The listing builds one solid part. Answer for the finished solid, in the listing's coordinates (mm). A direction names the side the tool comes from. Round coordinates to 2 decimals unless told otherwise and drop trailing zeros. Write each loop counter-clockwise with the first axis right and the second up, starting at its lowest first coordinate (ties: lowest second). Pieces come first, ordered by that corner, then holes. Notation, with made-up numbers: M 43.5,5 L 73.5,5 A10 cw 73.5,19 Z; hole C 60,-9.5 d6. An arc over 180 degrees is marked long. Put each result on its own line as item: value. Start each with the question number.
```python
from build123d import *

# Parameters (mm, degrees)
SKETCH1_W               = 21.8
SKETCH1_H               = 39
BOSS_EXTRUDE1_DEPTH     = 3
BOSS_EXTRUDE2_DEPTH     = 3
BOSS_EXTRUDE4_DEPTH     = 21
SKETCH4_W               = 21.8
SKETCH4_H               = 39
BOSS_EXTRUDE5_DEPTH     = 2
CUT_EXTRUDE1_DEPTH      = 50.807730324
CUT_EXTRUDE1_DEPTH_BACK = 50.807730324
SKETCH5_W               = 14
SKETCH5_H               = 20
BOSS_EXTRUDE6_DEPTH     = 5
SKETCH7_W               = 14.6
SKETCH7_H               = 1.5
CUT_EXTRUDE2_DEPTH      = 2
SKETCH8_W               = 16.04420395
SKETCH8_H               = 34.30198165
CUT_EXTRUDE3_DEPTH      = 35.279148181
SKETCH9_W               = 16.04420395
SKETCH9_H               = 34.30198165
CUT_EXTRUDE4_DEPTH      = 2
SKETCH10_W              = 2.1
SKETCH10_H              = 1.5
CUT_EXTRUDE5_DEPTH      = 2
SKETCH11_W              = 2.1
SKETCH11_H              = 1.5
CUT_EXTRUDE6_DEPTH      = 2
SKETCH13_W              = 18.8
SKETCH13_H              = 1.5
CUT_EXTRUDE7_DEPTH      = 3
FILLET3_R               = 5
FILLET4_R               = 5
SKETCH17_W              = 1.5
SKETCH17_H              = 16
BOSS_EXTRUDE8_DEPTH     = 2
FILLET5_R               = 5
BOSS_EXTRUDE9_DEPTH     = 5
SKETCH24_R              = 2.25
BOSS_EXTRUDE10_DEPTH    = 8
BOSS_EXTRUDE11_START    = 8
SKETCH25_R              = 2.25
BOSS_EXTRUDE11_DEPTH    = 8
FILLET7_R               = 5


with BuildPart() as part:
    # Sketch1 → Boss-Extrude1 (new body)
    with BuildSketch(Plane.XY):
        Rectangle(SKETCH1_W, SKETCH1_H)
    extrude(amount=BOSS_EXTRUDE1_DEPTH)

    # Sketch2 → Boss-Extrude2 (add)
    with BuildSketch(Plane.XY.offset(3)):
        Polygon((-10.9, 19.5), (-9.4, 19.5), (-9.4, -18), (9.4, -18), (9.4, 19.5), (10.9, 19.5), (10.9, -19.5), (-10.9, -19.5), align=None)
    extrude(amount=BOSS_EXTRUDE2_DEPTH)

    # Sketch3 → Boss-Extrude4 (add)
    with BuildSketch(Plane.XY.offset(6)):
        Polygon((-9.4, -18), (-10.9, -18), (-10.9, -19.5), (10.9, -19.5), (10.9, -18), align=None)
    extrude(amount=BOSS_EXTRUDE4_DEPTH)

    # Sketch4 → Boss-Extrude5 (add)
    with BuildSketch(Plane.XY.offset(27)):
        Rectangle(SKETCH4_W, SKETCH4_H)
    extrude(amount=BOSS_EXTRUDE5_DEPTH)

    # Sketch5 → Cut-Extrude1 (cut, two sides: drawn at the far end of the back side and taken through both)
    with BuildSketch(Plane.XZ.offset(19.5).offset(-CUT_EXTRUDE1_DEPTH_BACK)):
        with Locations((0, 14.5)):
            Rectangle(SKETCH5_W, SKETCH5_H)
    extrude(amount=CUT_EXTRUDE1_DEPTH + CUT_EXTRUDE1_DEPTH_BACK, mode=Mode.SUBTRACT)

    # Sketch6 → Boss-Extrude6 (add)
    with BuildSketch(Plane(origin=(0, 0, 27), x_dir=(-1, 0, 0), z_dir=(0, 0, -1))):
        Polygon((-9.4, -18), (-9.4, 18), (9.4, 18), (9.4, -18), (10.9, -18), (10.9, 19.5), (-10.9, 19.5), (-10.9, -18), align=None)
    extrude(amount=BOSS_EXTRUDE6_DEPTH)

    # Sketch7 → Cut-Extrude2 (cut)
    with BuildSketch(Plane(origin=(0, 0, 22), x_dir=(-1, 0, 0), z_dir=(0, 0, -1))):
        with Locations((0, 18.75)):
            Rectangle(SKETCH7_W, SKETCH7_H)
    extrude(amount=-CUT_EXTRUDE2_DEPTH, mode=Mode.SUBTRACT)

    # Sketch8 → Cut-Extrude3 (cut, through all)
    with BuildSketch(Plane.XY.offset(3)):
        Rectangle(SKETCH8_W, SKETCH8_H)
    extrude(amount=-CUT_EXTRUDE3_DEPTH, mode=Mode.SUBTRACT)

    # Sketch9 → Cut-Extrude4 (cut)
    with BuildSketch(Plane(origin=(0, 0, 27), x_dir=(-1, 0, 0), z_dir=(0, 0, -1))):
        Rectangle(SKETCH9_W, SKETCH9_H)
    extrude(amount=-CUT_EXTRUDE4_DEPTH, mode=Mode.SUBTRACT)

    # Sketch10 → Cut-Extrude5 (cut)
    with BuildSketch(Plane(origin=(0, 0, 22), x_dir=(-1, 0, 0), z_dir=(0, 0, -1))):
        with Locations((8.35, 18.75)):
            Rectangle(SKETCH10_W, SKETCH10_H)
    extrude(amount=-CUT_EXTRUDE5_DEPTH, mode=Mode.SUBTRACT)

    # Sketch11 → Cut-Extrude6 (cut)
    with BuildSketch(Plane(origin=(0, 0, 22), x_dir=(-1, 0, 0), z_dir=(0, 0, -1))):
        with Locations((-8.35, 18.75)):
            Rectangle(SKETCH11_W, SKETCH11_H)
    extrude(amount=-CUT_EXTRUDE6_DEPTH, mode=Mode.SUBTRACT)

    # Sketch13 → Cut-Extrude7 (cut)
    with BuildSketch(Plane(origin=(0, 0, 24), x_dir=(-1, 0, 0), z_dir=(0, 0, -1))):
        with Locations((0, 18.75)):
            Rectangle(SKETCH13_W, SKETCH13_H)
    extrude(amount=-CUT_EXTRUDE7_DEPTH, mode=Mode.SUBTRACT)

    # Fillet3
    fillet3_edges = [part.edges().sort_by_distance(p)[0] for p in [
        (8.022101975, 17.150990825, 1.5),
        (8.022101975, -17.150990825, 1.5),
        (-8.022101975, -17.150990825, 1.5),
        (-8.022101975, 17.150990825, 1.5),
        (-8.022101975, -17.150990825, 28),
        (8.022101975, -17.150990825, 28),
    ]]
    fillet(fillet3_edges, radius=FILLET3_R)

    # Fillet4
    fillet4_edges = [part.edges().sort_by_distance(p)[0] for p in [
        (-8.022101975, 17.150990825, 28),
        (8.022101975, 17.150990825, 28),
    ]]
    fillet(fillet4_edges, radius=FILLET4_R)

    # Sketch17 → Boss-Extrude8 (add)
    with BuildSketch(Plane(origin=(0, -18, 0), x_dir=(1, 0, 0), z_dir=(0, 1, 0))):
        with Locations((-10.15, -14)):
            Rectangle(SKETCH17_W, SKETCH17_H)
        with Locations((10.15, -14)):
            Rectangle(SKETCH17_W, SKETCH17_H)
    extrude(amount=BOSS_EXTRUDE8_DEPTH)

    # Fillet5
    fillet5_edges = [part.edges().sort_by_distance(p)[0] for p in [
        (-10.15, -16, 22),
        (-10.15, -16, 6),
        (10.15, -16, 6),
        (10.15, -16, 22),
        (7, -18.75, 24.5),
        (7, -18.75, 4.5),
        (-7, -18.75, 4.5),
        (-7, -18.75, 24.5),
    ]]
    fillet(fillet5_edges, radius=FILLET5_R)

    # Sketch19 → Boss-Extrude9 (add)
    with BuildSketch(Plane.XY.offset(29)):
        Polygon((-10.9, 19.5), (-10.9, -19.5), (-8.022101975, -19.5), (-8.022101975, -12.150990825), (-8.022101975, 12.150990825), (-8.022101975, 19.5), align=None)
        Polygon((8.022101975, 12.150990825), (8.022101975, 19.5), (10.9, 19.5), (10.9, -19.5), (8.022101975, -19.5), align=None)
    extrude(amount=BOSS_EXTRUDE9_DEPTH)

    # Sketch24 → Boss-Extrude10 (add)
    with BuildSketch(Plane.ZY.offset(10.9)):
        with Locations(Location((31, 8.15, 0), (0, 0, 180))):
            Circle(SKETCH24_R)
        with Locations(Location((31, 0.15, 0), (0, 0, 180))):
            Circle(SKETCH24_R)
        with Locations(Location((31, -7.85, 0), (0, 0, 180))):
            Circle(SKETCH24_R)
    extrude(amount=BOSS_EXTRUDE10_DEPTH)

    # Sketch25 → Boss-Extrude11 (add)
    with BuildSketch(Plane(origin=(10.9, 0, 0), x_dir=(0, 0, -1), z_dir=(1, 0, 0)).offset(BOSS_EXTRUDE11_START)):
        with Locations((-31, 8.15)):
            Circle(SKETCH25_R)
        with Locations((-31, 0.15)):
            Circle(SKETCH25_R)
        with Locations((-31, -7.85)):
            Circle(SKETCH25_R)
    extrude(amount=-BOSS_EXTRUDE11_DEPTH)

    # Fillet7
    fillet7_edges = [part.edges().sort_by_distance(p)[0] for p in [
        (-9.461050988, -19.5, 34),
        (9.461050988, -19.5, 34),
        (-10.15, 19.5, 6),
        (9.461050988, 19.5, 34),
        (-9.461050988, 19.5, 34),
    ]]
    fillet(fillet7_edges, radius=FILLET7_R - 0.0001)  # a hair under: the kernel refuses the full size


solid = part.part
```
Item 1: Section D-D (x = 4.5) is taken. Give the vertices of the cut face in (y, z), and give its area (3 significant figures).
Item 2: Which of the six approach directions +Z, -Z, +X, -X, +Y, -Y give full straight-line access (tool end or side, diameter ignored) to faces 4 (the cylindrical face through (5.5, -18.76, 5.93)), 5 (the flat face through (-10, 2, 6)), 6 (the cylindrical face through (6.596, -15.647, 1.479)), 7 (the flat face through (-8.4, 4.7, 3))?
Item 3: Consider line 1 along X through (y, z) = (-4, 24.5); line 2 along X through (y, z) = (-3.5, 28); line 3 along Z through (x, y) = (9, -9.5). Determine where each line is inside the solid, lowest interval first. Write a range as [from, to].
Item 4: Section B-B (x = 0) is taken. Give the vertices of the cut face in (y, z).
Item 5: Section C-C (z = 13.5) is taken. Give the vertices of the cut face in (x, y).
Item 6: Section A-A (y = -7.85) is taken. Count the separate pieces of the cut face and the enclosed holes in it, and give its area (3 significant figures).
Item 7: Flat-ended cylindrical pins translate along their axes: pin 1 (2.5 mm diameter, centred on y = 4.5, z = 1, fed in from +X); pin 2 (5 mm diameter, centred on y = -12.5, z = 13, fed in from -X); pin 3 (0.8 mm diameter, centred on y = -18.5, z = 14, fed in from -X); pin 4 (1.6 mm diameter, centred on x = 10, z = 15, fed in from +Y). Find the tip coordinate at first contact, or state that the pin passes through.
Item 8: Determine the mould class of faces 1 (the flat face through (0, 17.151, 2)), 2 (the flat face through (10, -16, 14)), 3 (the cylindrical face through (-14.84, -6.99, 28.92)) for opening direction Z: released by +Z, released by -Z, zero draft, split by the parting line, or undercut.
Output values:
1. outline: M -19.5,0 L -16.93,0 L -16.93,3 L -18,3 L -18,5.17 L -19.5,5.17 Z; M -19.5,23.83 L -18,23.83 L -18,27 L -16.93,27 L -16.93,29 L -19.5,29 Z; M 16.93,0 L 19.5,0 L 19.5,1 A5 ccw 19.08,3 L 16.93,3 Z; M 16.93,27 L 19.5,27 L 19.5,29 L 16.93,29 Z
1. area: 33.5 mm^2
2. face 4: +Y, -Y
2. face 5: +X, -X, +Y
2. face 6: +Z, -Z
2. face 7: +Y
3. line 1: x = [-10.9, -9.4], [9.4, 10.9]
3. line 2: x = [-10.9, -8.02], [8.02, 10.9]
3. line 3: z = [0, 3], [27, 34]
4. outline: M -19.5,0 L -17.15,0 L -17.15,3 L -18,3 L -18,4.5 L -19.5,4.5 Z; M -19.5,24.5 L -18,24.5 L -18,27 L -17.15,27 L -17.15,29 L -19.5,29 Z; M 17.15,0 L 19.5,0 L 19.5,1 A5 ccw 19.08,3 L 17.15,3 Z; M 17.15,27 L 19.5,27 L 19.5,29 L 17.15,29 Z
5. outline: M -10.9,-19.5 L -7,-19.5 L -7,-18 L -9.4,-18 L -9.4,-16 L -10.9,-16 Z; M 7,-19.5 L 10.9,-19.5 L 10.9,-16 L 9.4,-16 L 9.4,-18 L 7,-18 Z
6. separate pieces: 4
6. enclosed holes: 0
6. area: 154 mm^2
7. pin 1: stops at x = 10.9
7. pin 2: passes through
7. pin 3: stops at x = -10.9
7. pin 4: stops at y = -16
8. face 1: zero draft
8. face 2: undercut
8. face 3: split by the parting line
